from build123d import *

# Parameters (mm, degrees)
F0_R      = 6
F1_DEPTH  = 3
F2_R      = 5.75
F3_DEPTH  = 1.15
F4_R      = 6
F4_R_2    = 5.75
F5_DEPTH  = 16
F6_R      = 7.5
F6_R_2    = 6
F7_DEPTH  = 667
F8_R      = 6
F9_DEPTH  = 15
F10_R     = 5.95
F11_DEPTH = 2
F12_R     = 5.95
F13_DEPTH = 3
F14_R     = 5
F15_DEPTH = 15
F16_SIZE  = 1


with BuildPart() as f1:
    # F0 (on Top) → F1 (new body)
    with BuildSketch(Plane.XY):
        Circle(F0_R)
    extrude(amount=F1_DEPTH)

    # F2 (on face) → F3 (join)
    with BuildSketch(Plane.XY.offset(3)):
        Circle(F2_R)
    extrude(amount=F3_DEPTH)

    # F4 (on face) → F5 (join)
    with BuildSketch(Plane.XY.offset(4.15)):
        Circle(F4_R)
        Circle(F4_R_2, mode=Mode.SUBTRACT)
        Circle(F4_R_2)
    extrude(amount=F5_DEPTH)

    # F6 (on face) → F7 (join)
    with BuildSketch(Plane.XY.offset(20.15)):
        Circle(F6_R)
        Circle(F6_R_2, mode=Mode.SUBTRACT)
        Circle(F6_R_2)
    extrude(amount=F7_DEPTH)

    # F8 (on face) → F9 (join)
    with BuildSketch(Plane.XY.offset(687.15)):
        Circle(F8_R)
    extrude(amount=F9_DEPTH)

    # F10 (on face) → F11 (join)
    with BuildSketch(Plane.XY.offset(702.15)):
        Circle(F10_R)
    extrude(amount=F11_DEPTH)

    # F12 (on face) → F13 (join)
    with BuildSketch(Plane.XY.offset(704.15)):
        Circle(F12_R)
    extrude(amount=F13_DEPTH)

    # F14 (on face) → F15 (join)
    with BuildSketch(Plane.XY.offset(707.15)):
        Circle(F14_R)
    extrude(amount=F15_DEPTH)

    # F16
    f16_edges = [f1.edges().sort_by_distance(p)[0] for p in [
        (-5, 0, 722.15),
        (-6, 0, 0),
    ]]
    chamfer(f16_edges, length=F16_SIZE)


solid = f1.part
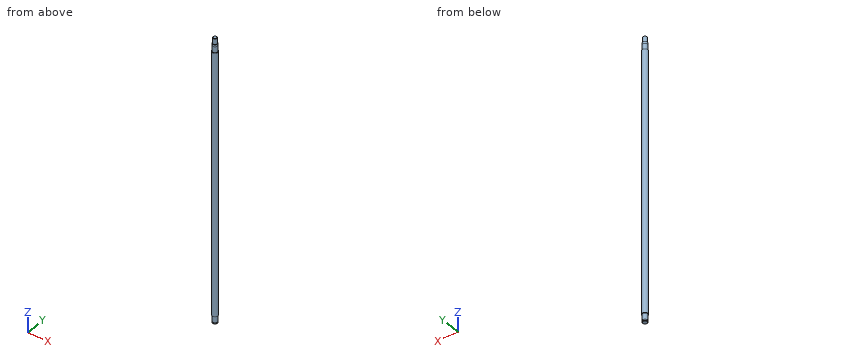
Source: CAD feature listing. Evaluate the final solid. Frame: model axes, mm. Coordinates: 2 decimals unless noted, no trailing zeros. Order: outer loops, then holes, each group sorted by start corner. A loop starts at its lowest first (then second) coordinate and runs counter-clockwise, first axis right, second up.
Item 1: Cut plane C-C (z = 47.5). Return loops of the section in (x, y).
Output values:
outline: circle Ø15 at (0, 0)
Item 2: Material intervals for line 1 (X direction, y = -4.5, z = 305); line 2 (Z direction, x = -4.25, y = 4.75); line 3 (X direction, y = 0.75, z = 431), sorted ascending.
Output values:
line 1: x = -6 to 6
line 2: z = 20.15 to 687.15
line 3: x = -7.46 to 7.46
Item 3: First-contact query: P1, Ø1, axis at x = -3.5, y = 4.5, coming from the -Z side; P2, Ø7.5, axis at x = 1, y = 3.5, coming from the -Z side; P3, Ø1, axis at y = 2.5, z = 492, coming from the -X side; P4, Ø2, axis at x = 2.5, z = 538, coming from the +Y side. Flat tips, straight axial feed; report the tip coordinate or a pass-through.
Output values:
P1: stops at z = 0.2
P2: stops at z = 0
P3: stops at x = -7.23
P4: stops at y = 7.35
